```python
from build123d import *

# Parameters (mm, degrees)
SKETCH_1_W          = 130
SKETCH_1_H          = 95
EXTRUDE_1_DEPTH     = 3
SKETCH_3_R          = 1.5
CUT_EXTRUDE_2_DEPTH = 10
SKETCH_4_R          = 1.5
CUT_EXTRUDE_3_DEPTH = 10


with BuildPart() as part:
    # 草图1 → 凸台-拉伸1 (new body)
    with BuildSketch(Plane.XY):
        Rectangle(SKETCH_1_W, SKETCH_1_H)
    extrude(amount=EXTRUDE_1_DEPTH)

    # 草图3 → 切除-拉伸2 (cut)
    with BuildSketch(Plane(origin=(0, 0, 0), x_dir=(-1, 0, 0), z_dir=(0, 0, -1))):
        with Locations((-57.767112616, -26.5)):
            Circle(SKETCH_3_R)
        with Locations((-41.767112616, -26.5)):
            Circle(SKETCH_3_R)
        with Locations((42.232887384, -26.5)):
            Circle(SKETCH_3_R)
        with Locations((58.232887384, -26.5)):
            Circle(SKETCH_3_R)
    extrude(amount=-CUT_EXTRUDE_2_DEPTH, mode=Mode.SUBTRACT)

    # 草图4 → 切除-拉伸3 (cut)
    with BuildSketch(Plane(origin=(0, 0, 0), x_dir=(-1, 0, 0), z_dir=(0, 0, -1))):
        with Locations((-46.767112616, 42.5)):
            Circle(SKETCH_4_R)
        with Locations((-46.767112616, 22.5)):
            Circle(SKETCH_4_R)
        with Locations((47.232887384, 42.5)):
            Circle(SKETCH_4_R)
        with Locations((47.232887384, 22.5)):
            Circle(SKETCH_4_R)
    extrude(amount=-CUT_EXTRUDE_3_DEPTH, mode=Mode.SUBTRACT)


solid = part.part
```
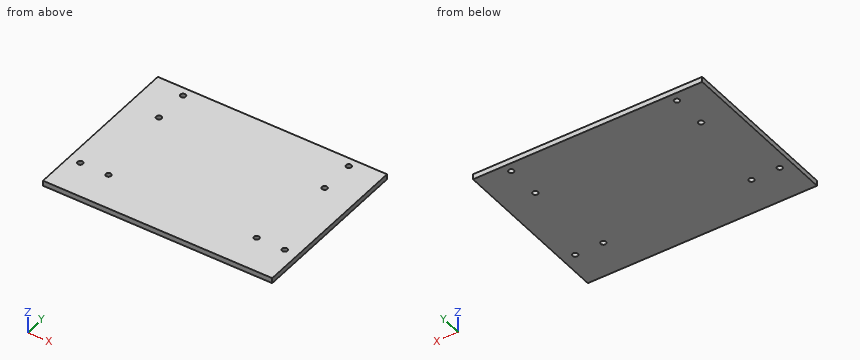
Geometry: final body of the model. Coordinates: model frame, mm. Give positions to 0.01 mm unless a question says otherwise; leave off trailing zeros. Order: outer loops, then holes, each group sorted by start corner. A loop starts at its lowest first (then second) coordinate and runs counter-clockwise, first axis right, second up. Notation, with made-up numbers: (44, 53.5) -> (69, 53.5) arc R17 cw to (69, 70.5) -> close; hole circle Ø9 at (52, 48). An arc over 180 degrees is marked (long way). Write each question's results on one line, items separated by ' | '. Start each with the question number.
1) Section A-A (y = 22.5). Return loops of the section in (x, z), then the cut area to 3 significant figures.
2) Section B-B (y = -26.5). Return loops of the section in (x, z).
3) Line query: line 1 (Y direction, x = 43, z = 1.8); line 2 (Y direction, x = -46.5, z = 1.65). Output: solid intervals per line, ascending. Write a range as from..to.
4) First-contact query: pin 1 (3.5 mm diameter, centred on x = 46.77, y = 42.5, fed in from +Z). Flat tip, straight axial feed; report the tip coordinate or a pass-through.
Calculated:
1) outline: (-65, 0) -> (-48.73, 0) -> (-48.73, 3) -> (-65, 3) -> close; (-45.73, 0) -> (45.27, 0) -> (45.27, 3) -> (-45.73, 3) -> close; (48.27, 0) -> (65, 0) -> (65, 3) -> (48.27, 3) -> close | area: 372 mm2
2) outline: (-65, 0) -> (-59.73, 0) -> (-59.73, 3) -> (-65, 3) -> close; (-56.73, 0) -> (-43.73, 0) -> (-43.73, 3) -> (-56.73, 3) -> close; (-40.73, 0) -> (40.27, 0) -> (40.27, 3) -> (-40.73, 3) -> close; (43.27, 0) -> (56.27, 0) -> (56.27, 3) -> (43.27, 3) -> close; (59.27, 0) -> (65, 0) -> (65, 3) -> (59.27, 3) -> close
3) line 1: -47.5..-27.35, -25.65..47.5 | line 2: -47.5..21.19, 23.81..41.19, 43.81..47.5
4) pin 1: z = 3
